from build123d import *

# Parameters (mm, degrees)
BOSS_EXTRUDE1_DEPTH = 1.9558
SKETCH2_W           = 11.1506
SKETCH2_H           = 23.3426
BOSS_EXTRUDE2_DEPTH = 2.5019
SKETCH3_W           = 15.1892
SKETCH3_H           = 33.5026
BOSS_EXTRUDE3_DEPTH = 20.32
SKETCH4_R           = 12.85875
CUT_EXTRUDE1_DEPTH  = 40.489177087
SKETCH5_W           = 11.3792
SKETCH5_H           = 2.54
CUT_EXTRUDE2_DEPTH  = 44.289434312
FILLET1_R           = 1.27
SKETCH6_W           = 7.5692
SKETCH6_H           = 13.97
CUT_EXTRUDE3_DEPTH  = 1.27
SKETCH7_W           = 7.5692
SKETCH7_H           = 13.97
CUT_EXTRUDE4_DEPTH  = 1.27


with BuildPart() as part:
    # Sketch1 → Boss-Extrude1 (new body)
    with BuildSketch(Plane(origin=(0, 0, 0), x_dir=(1, 0, 0), z_dir=(0, 1, 0))):
        with BuildLine():
            Line((2.1971, 0), (12.9921, 0))
            ThreePointArc((12.9921, 0), (14.545684309, -0.643515691), (15.1892, -2.1971))
            Line((15.1892, -2.1971), (15.1892, -21.1455))
            ThreePointArc((15.1892, -21.1455), (14.545684309, -22.699084309), (12.9921, -23.3426))
            Line((12.9921, -23.3426), (2.1971, -23.3426))
            ThreePointArc((2.1971, -23.3426), (0.643515691, -22.699084309), (0, -21.1455))
            Line((0, -21.1455), (0, -2.1971))
            ThreePointArc((0, -2.1971), (0.643515691, -0.643515691), (2.1971, 0))
        make_face()
    extrude(amount=BOSS_EXTRUDE1_DEPTH)

    # Sketch2 → Boss-Extrude2 (add)
    with BuildSketch(Plane.XZ):
        with Locations((7.5946, 11.6713)):
            Rectangle(SKETCH2_W, SKETCH2_H)
    extrude(amount=BOSS_EXTRUDE2_DEPTH)

    # Sketch3 → Boss-Extrude3 (add)
    with BuildSketch(Plane.XZ.offset(2.5019)):
        with Locations((7.5946, 11.6713)):
            Rectangle(SKETCH3_W, SKETCH3_H)
    extrude(amount=BOSS_EXTRUDE3_DEPTH)

    # Sketch4 → Cut-Extrude1 (cut, through all)
    with BuildSketch(Plane(origin=(15.1892, 0, 0), x_dir=(0, 0, -1), z_dir=(1, 0, 0))):
        with Locations((-11.6713, -22.8219)):
            Circle(SKETCH4_R)
    extrude(amount=-CUT_EXTRUDE1_DEPTH, mode=Mode.SUBTRACT)

    # Sketch5 → Cut-Extrude2 (cut, through all)
    with BuildSketch(Plane.XY.offset(28.4226)):
        with Locations((7.5946, -7.5819)):
            Rectangle(SKETCH5_W, SKETCH5_H)
    extrude(amount=-CUT_EXTRUDE2_DEPTH, mode=Mode.SUBTRACT)

    # Fillet1
    fillet1_edges = [part.edges().sort_by_distance(p)[0] for p in [
        (13.2842, -8.8519, 11.6713),
        (13.2842, -6.3119, 11.6713),
        (1.905, -6.3119, 11.6713),
        (1.905, -8.8519, 11.6713),
    ]]
    fillet(fillet1_edges, radius=FILLET1_R - 0.0001)  # a hair under: the kernel refuses the full size

    # Sketch6 → Cut-Extrude3 (cut)
    with BuildSketch(Plane(origin=(0, 0, -5.08), x_dir=(-1, 0, 0), z_dir=(0, 0, -1))):
        with Locations((-7.5946, -15.8369)):
            Rectangle(SKETCH6_W, SKETCH6_H)
    extrude(amount=-CUT_EXTRUDE3_DEPTH, mode=Mode.SUBTRACT)

    # Sketch7 → Cut-Extrude4 (cut)
    with BuildSketch(Plane.XY.offset(28.4226)):
        with Locations((7.5946, -15.8369)):
            Rectangle(SKETCH7_W, SKETCH7_H)
    extrude(amount=-CUT_EXTRUDE4_DEPTH, mode=Mode.SUBTRACT)


solid = part.part
CAD build for the part. Positions are in the model's coordinates, mm. A direction names the side the tool comes from. Coordinates: 2 decimals unless noted, no trailing zeros. Order: outer loops, then holes, each group sorted by start corner. A loop starts at its lowest first (then second) coordinate and runs counter-clockwise, first axis right, second up.
Item 1: Pin check, flat tips, straight feed: pin 1 Ø1 at (x, z) = (14.5, 7.5) entering from -Y; pin 2 Ø1.3 at (x, y) = (5.5, 0.5) entering from -Z; pin 3 Ø1 at (x, z) = (8.5, 13) entering from -Y. Stop position of each tip, or through.
Check sheet entries:
pin 1: stops at y = -10.84
pin 2: stops at z = 0
pin 3: stops at y = -10.09
Item 2: Band-saw the part on D-D on y = -14. List the corners of the cut face in (x, z), plus the area to 3 significant figures.
Check sheet entries:
outline: (0, -5.08) - (3.81, -5.08) - (3.81, -3.81) - (11.38, -3.81) - (11.38, -5.08) - (15.19, -5.08) - (15.19, 2.32) - (0, 2.32) - close; (0, 21.03) - (15.19, 21.03) - (15.19, 28.42) - (11.38, 28.42) - (11.38, 27.15) - (3.81, 27.15) - (3.81, 28.42) - (0, 28.42) - close
area: 205 mm2
Item 3: Band-saw the part on B-B on y = -9.5. List the corners of the cut face in (x, z), plus the area to 3 significant figures.
Check sheet entries:
outline: (0, -5.08) - (3.81, -5.08) - (3.81, -3.81) - (11.38, -3.81) - (11.38, -5.08) - (15.19, -5.08) - (15.19, 28.42) - (11.38, 28.42) - (11.38, 27.15) - (3.81, 27.15) - (3.81, 28.42) - (0, 28.42) - close
area: 490 mm2
Item 4: 3-axis set-ups, long thin cutter, end or side, ignore diameter. For faces 1 (the face through (1, 0, 12)), 2 (the face through (14.5, 1, 0.6)), 3 (the face through (0.661, 0.964, 22.716)): which of +Z, -Z, +X, -X, +Y, -Y reach the whole face in a straight line?
Check sheet entries:
face 1: +Z, -Z, -X
face 2: -Z, +X, +Y
face 3: +Z, -X, +Y
Item 5: Band-saw the part on A-A on x = 4.5. List the corners of the cut face in (y, z).
Check sheet entries:
outline: (-22.82, -3.81) - (-8.85, -3.81) - (-8.85, 27.15) - (-22.82, 27.15) - (-22.82, 24.53) arc R12.86 cw to (-22.82, -1.19) - close; (-6.31, -5.08) - (-2.5, -5.08) - (-2.5, 0) - (1.96, 0) - (1.96, 23.34) - (-2.5, 23.34) - (-2.5, 28.42) - (-6.31, 28.42) - close
Item 6: Two-plate mould, pull along X, no slides. Class faces 4 (the face through (0.63, 0.96, 0.66)), 5 (the face through (11.379, -16, 28)), 6 (the face through (8, 0, 0)): +X half, -X half, draft (parallel to the pull), parting line (faces both ways), or undercut.
Check sheet entries:
face 4: -X half
face 5: undercut
face 6: draft
Item 7: Drill centre lines: L1, parallel to X at y = -7.5, z = 3.5; L2, parallel to Z at x = 4, y = -0.75; L3, parallel to Y at x = 7, z = 9.5. Where is each one in solid material? Low to high.
Check sheet entries:
L1: x = 0 to 1.91, 13.28 to 15.19
L2: z = 0 to 23.34
L3: y = -10.15 to -8.85, -6.31 to 1.96
